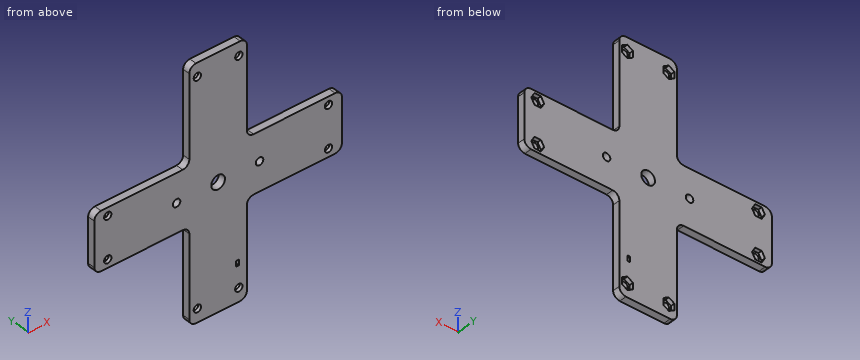
Autodesk Inventor part; units mm, degrees
ref_plane "YZ Plane" through (0, 0, 0) normal (1, 0, 0) x (0, 1, 0)
ref_plane "XZ Plane" through (0, 0, 0) normal (0, 1, 0) x (-1, 0, 0)
ref_plane "XY Plane" through (0, 0, 0) normal (0, 0, 1) x (1, 0, 0)
sketch "Sketch1" plane through (0, 0, 0) normal (0, 1, 0) x (1, 0, 0)
  circle A0 centre (0, 0) radius 2.25
  circle A1 centre (31, 0) radius 2.25
  circle A2 centre (0, 31) radius 2.25
  circle A3 centre (31, 31) radius 2.25
  circle A4 centre (15.5, 15.5) radius 5.125
  line L0 (-6, 37) -> (37, 37)
  line L1 (37, 37) -> (37, -6)
  line L2 (37, -6) -> (-6, -6)
  line L3 (-6, -6) -> (-6, 37)
  line L4 (-6, 37) -> (37, -6) construction
  line L5 (37, 37) -> (-6, -6) construction
  line L6 (-6, -6) -> (37, -6)
  circle A5 centre (0, 98) radius 2.75
  circle A6 centre (31, 98) radius 2.75
  line L7 (-6, 37) -> (37, 37)
  line L8 (37, 37) -> (37, 108)
  line L9 (37, 108) -> (-6, 108)
  line L10 (-6, 108) -> (-6, 37)
  line L11 (15.5, 15.5) -> (22.827, 15.5)
  line L12 (13, 103) -> (18, 103)
  line L13 (15.5, 103) -> (15.5, 96.4439)
  arc A7 (0, 95.25) -> (0, 100.75) centre (0, 98) ccw
  circle A8 centre (-15.5, 15.5) radius 2.7971
  circle A9 centre (46.5, 15.5) radius 2.7971
  line L14 (0, 93.4736) -> (-3.92, 95.7368)
  line L15 (-3.92, 95.7368) -> (-3.92, 100.2632)
  line L16 (-3.92, 100.2632) -> (0, 102.5264)
  line L17 (0, 102.5264) -> (3.92, 100.2632)
  line L18 (3.92, 100.2632) -> (3.92, 95.7368)
  line L19 (3.92, 95.7368) -> (0, 93.4736)
  line L20 (4.17, 100.4076) -> (0, 102.8151)
  line L21 (0, 102.8151) -> (-4.17, 100.4076)
  line L22 (-4.17, 100.4076) -> (-4.17, 95.5924)
  line L23 (-4.17, 95.5924) -> (0, 93.1849)
  line L24 (0, 93.1849) -> (4.17, 95.5924)
  line L25 (4.17, 95.5924) -> (4.17, 100.4076)
  circle A10 centre (31, 98) radius 2.75
  circle A11 centre (31, 98) radius 2.75
  arc A12 (31, 100.75) -> (31, 95.25) centre (31, 98) ccw
  line L26 (31, 93.4736) -> (34.92, 95.7368)
  line L27 (34.92, 95.7368) -> (34.92, 100.2632)
  line L28 (34.92, 100.2632) -> (31, 102.5264)
  line L29 (31, 102.5264) -> (27.08, 100.2632)
  line L30 (27.08, 100.2632) -> (27.08, 95.7368)
  line L31 (27.08, 95.7368) -> (31, 93.4736)
  line L32 (26.83, 100.4076) -> (31, 102.8151)
  line L33 (31, 102.8151) -> (35.17, 100.4076)
  line L34 (35.17, 100.4076) -> (35.17, 95.5924)
  line L35 (35.17, 95.5924) -> (31, 93.1849)
  line L36 (31, 93.1849) -> (26.83, 95.5924)
  line L37 (26.83, 95.5924) -> (26.83, 100.4076)
  line L38 (-64.7368, -3.92) -> (-69.2632, -3.92)
  line L39 (-69.4076, -4.17) -> (-64.5924, -4.17)
  line L40 (-69.2632, -3.92) -> (-71.5264, 0)
  line L41 (-71.8151, 0) -> (-69.4076, -4.17)
  circle A13 centre (-67, 31) radius 2.75
  line L42 (-72, 13) -> (-72, 18)
  line L43 (-69.2632, 27.08) -> (-64.7368, 27.08)
  line L44 (-64.7368, 34.92) -> (-69.2632, 34.92)
  line L45 (-64.5924, 26.83) -> (-69.4076, 26.83)
  circle A14 centre (-67, 31) radius 2.75
  circle A15 centre (-67, 31) radius 2.75
  arc A16 (-69.75, 31) -> (-64.25, 31) centre (-67, 31) ccw
  line L46 (-72, 15.5) -> (-65.4439, 15.5)
  line L47 (-69.2632, 34.92) -> (-71.5264, 31)
  line L48 (-71.8151, 31) -> (-69.4076, 35.17)
  line L49 (-69.4076, 35.17) -> (-64.5924, 35.17)
  line L50 (-71.5264, 31) -> (-69.2632, 27.08)
  line L51 (-69.4076, 26.83) -> (-71.8151, 31)
  line L52 (-62.4736, 0) -> (-64.7368, -3.92)
  line L53 (-64.5924, -4.17) -> (-62.1849, 0)
  circle A17 centre (-67, 0) radius 2.75
  arc A18 (-64.25, 0) -> (-69.75, 0) centre (-67, 0) ccw
  line L54 (-71.5264, 0) -> (-69.2632, 3.92)
  line L55 (-69.4076, 4.17) -> (-71.8151, 0)
  line L56 (-69.2632, 3.92) -> (-64.7368, 3.92)
  line L57 (-64.5924, 4.17) -> (-69.4076, 4.17)
  line L58 (-62.1849, 0) -> (-64.5924, 4.17)
  line L59 (-64.7368, 3.92) -> (-62.4736, 0)
  line L60 (-62.1849, 31) -> (-64.5924, 26.83)
  line L61 (-64.7368, 27.08) -> (-62.4736, 31)
  line L62 (-77, -6) -> (-6, -6)
  line L63 (-62.4736, 31) -> (-64.7368, 34.92)
  line L64 (-64.5924, 35.17) -> (-62.1849, 31)
  line L65 (-77, 37) -> (-77, -6)
  line L66 (-6, 37) -> (-77, 37)
  line L67 (34.92, -64.7368) -> (34.92, -69.2632)
  line L68 (35.17, -69.4076) -> (35.17, -64.5924)
  line L69 (34.92, -69.2632) -> (31, -71.5264)
  line L70 (31, -71.8151) -> (35.17, -69.4076)
  circle A19 centre (0, -67) radius 2.75
  line L71 (18, -72) -> (13, -72)
  line L72 (3.92, -69.2632) -> (3.92, -64.7368)
  line L73 (-3.92, -64.7368) -> (-3.92, -69.2632)
  line L74 (4.17, -64.5924) -> (4.17, -69.4076)
  circle A20 centre (0, -67) radius 2.75
  circle A21 centre (0, -67) radius 2.75
  arc A22 (0, -69.75) -> (0, -64.25) centre (0, -67) ccw
  line L75 (15.5, -72) -> (15.5, -65.4439)
  line L76 (-3.92, -69.2632) -> (0, -71.5264)
  line L77 (0, -71.8151) -> (-4.17, -69.4076)
  line L78 (-4.17, -69.4076) -> (-4.17, -64.5924)
  line L79 (0, -71.5264) -> (3.92, -69.2632)
  line L80 (4.17, -69.4076) -> (0, -71.8151)
  line L81 (31, -62.4736) -> (34.92, -64.7368)
  line L82 (35.17, -64.5924) -> (31, -62.1849)
  circle A23 centre (31, -67) radius 2.75
  arc A24 (31, -64.25) -> (31, -69.75) centre (31, -67) ccw
  line L83 (31, -71.5264) -> (27.08, -69.2632)
  line L84 (26.83, -69.4076) -> (31, -71.8151)
  line L85 (27.08, -69.2632) -> (27.08, -64.7368)
  line L86 (26.83, -64.5924) -> (26.83, -69.4076)
  line L87 (31, -62.1849) -> (26.83, -64.5924)
  line L88 (27.08, -64.7368) -> (31, -62.4736)
  line L89 (0, -62.1849) -> (4.17, -64.5924)
  line L90 (3.92, -64.7368) -> (0, -62.4736)
  line L91 (37, -77) -> (37, -6)
  line L92 (0, -62.4736) -> (-3.92, -64.7368)
  line L93 (-4.17, -64.5924) -> (0, -62.1849)
  line L94 (-6, -77) -> (37, -77)
  line L95 (-6, -6) -> (-6, -77)
  line L96 (95.7368, 34.92) -> (100.2632, 34.92)
  line L97 (100.4076, 35.17) -> (95.5924, 35.17)
  line L98 (100.2632, 34.92) -> (102.5264, 31)
  line L99 (102.8151, 31) -> (100.4076, 35.17)
  circle A25 centre (98, 0) radius 2.75
  line L100 (103, 18) -> (103, 13)
  line L101 (100.2632, 3.92) -> (95.7368, 3.92)
  line L102 (95.7368, -3.92) -> (100.2632, -3.92)
  line L103 (95.5924, 4.17) -> (100.4076, 4.17)
  circle A26 centre (98, 0) radius 2.75
  circle A27 centre (98, 0) radius 2.75
  arc A28 (100.75, 0) -> (95.25, 0) centre (98, 0) ccw
  line L104 (103, 15.5) -> (96.4439, 15.5)
  line L105 (100.2632, -3.92) -> (102.5264, 0)
  line L106 (102.8151, 0) -> (100.4076, -4.17)
  line L107 (100.4076, -4.17) -> (95.5924, -4.17)
  line L108 (102.5264, 0) -> (100.2632, 3.92)
  line L109 (100.4076, 4.17) -> (102.8151, 0)
  line L110 (93.4736, 31) -> (95.7368, 34.92)
  line L111 (95.5924, 35.17) -> (93.1849, 31)
  circle A29 centre (98, 31) radius 2.75
  arc A30 (95.25, 31) -> (100.75, 31) centre (98, 31) ccw
  line L112 (102.5264, 31) -> (100.2632, 27.08)
  line L113 (100.4076, 26.83) -> (102.8151, 31)
  line L114 (100.2632, 27.08) -> (95.7368, 27.08)
  line L115 (95.5924, 26.83) -> (100.4076, 26.83)
  line L116 (93.1849, 31) -> (95.5924, 26.83)
  line L117 (95.7368, 27.08) -> (93.4736, 31)
  line L118 (93.1849, 0) -> (95.5924, 4.17)
  line L119 (95.7368, 3.92) -> (93.4736, 0)
  line L120 (108, 37) -> (37, 37)
  line L121 (93.4736, 0) -> (95.7368, -3.92)
  line L122 (95.5924, -4.17) -> (93.1849, 0)
  line L123 (108, -6) -> (108, 37)
  line L124 (37, -6) -> (108, -6)
  point P0 (37, 37)
  point P1 (37, 37)
  point P2 (-3.5, 98)
  point P3 (34.5, 98)
  point P4 (-67, -3.5)
  point P5 (-67, 34.5)
  point P6 (34.5, -67)
  point P7 (-3.5, -67)
  point P8 (98, 34.5)
  point P9 (98, -3.5)
  point P10 (-6, -6)
  point P11 (-6, -6)
  point P12 (-6, -6)
  point P13 (-6, -6)
  point P14 (-6, -6)
  point P15 (37, 37)
  dimension "d3" = 4.5
  dimension "d5" = 31
  dimension "d6" = 10.25
  dimension "d8" = 43
  dimension "d23" = 5.5
  dimension "d24" = 31
  dimension "d25" = 31
  dimension "d27" = 6
  dimension "d28" = 10
  dimension "d71" = 62
  dimension "d72" = 31
  dimension "d73" = 7.84
  dimension "d74" = 0.25
  dimension "d81" = 82.5
  dimension "d84" = 360
extrude "Extrusion4" add sketch "Sketch1" against normal blind 5.5 contours A0 | A1 | A2 | A3 | L10 L9 L8 L0 | L0 L1 L2 L3 | L3 L62 L65 L66 | L120 L123 L124 L1 | L2 L91 L94 L95 | L14 L15 L16 L17 L18 L19 | L25 L24 L23 L22 L21 L20 | L31 L30 L29 L28 L27 L26 | L32 L33 L34 L35 L36 L37 | L38 L40 L54 L56 L59 L52 | L41 L55 L57 L58 L53 L39 | L50 L47 L44 L63 L61 L43 | L45 L51 L48 L49 L64 L60 | L67 L69 L83 L85 L88 L81 | L70 L84 L86 L87 L82 L68 | L79 L76 L73 L92 L90 L72 | L74 L80 L77 L78 L93 L89 | L96 L98 L112 L114 L117 L110 | L99 L113 L115 L116 L111 L97 | L108 L105 L102 L121 L119 L101 | L103 L109 L106 L107 L122 L118
fillet "Fillet4" radius 5 4 edges at (-6, -2.75, -37) (-6, -2.75, 6) (37, -2.75, 6) (37, -2.75, -37)
fillet "Fillet5" radius 5 8 edges at (37, -2.75, -108) (-6, -2.75, -108) (108, -2.75, 6) (108, -2.75, -37) (37, -2.75, 77) (-6, -2.75, 77) (-77, -2.75, 6) (-77, -2.75, -37)
extrude "Extrusion7" cut sketch "Sketch1" against normal blind 3 contours A5 | A6 | L14 L15 L16 L17 L18 L19 | L25 L24 L23 L22 L21 L20 | L31 L30 L29 L28 L27 L26 | L32 L33 L34 L35 L36 L37 | L38 L40 L54 L56 L59 L52 | L41 L55 L57 L58 L53 L39 | A13 | L50 L47 L44 L63 L61 L43 | L45 L51 L48 L49 L64 L60 | A17 | L67 L69 L83 L85 L88 L81 | L70 L84 L86 L87 L82 L68 | A19 | L79 L76 L73 L92 L90 L72 | L74 L80 L77 L78 L93 L89 | A23 | L96 L98 L112 L114 L117 L110 | L99 L113 L115 L116 L111 L97 | A25 | L108 L105 L102 L121 L119 L101 | L103 L109 L106 L107 L122 L118 | A29
sketch "Sketch6" plane through (0, 0, 0) normal (0, 1, 0) x (1, 0, 0)
  line L0 (31, 78) -> (29, 78)
  line L1 (29, 78) -> (29, 82)
  line L2 (29, 82) -> (31, 82)
  line L3 (31, 82) -> (31, 78)
  line L4 (37, 42) -> (37, 103)
  line L5 (32, 108) -> (-1, 108)
  circle A0 centre (31, 98) radius 2.75
  point P0 (0, 0)
  dimension "d86" = 2
  dimension "d87" = 4
  dimension "d88" = 6
  dimension "d92" = 16
extrude "Extrusion8" cut sketch "Sketch6" against normal through all contours L0 L1 L2 L3
properties part number "motor_holder"
Source: CAD feature listing. Evaluate the final solid. Frame: model axes, mm. Round coordinates to 2 decimals unless told otherwise and drop trailing zeros. Write each loop counter-clockwise with the first axis right and the second up, starting at its lowest first coordinate (ties: lowest second). Pieces come first, ordered by that corner, then holes. Notation, with made-up numbers: (-4, -0.5) - (3, -0.5) arc R19 ccw to (3, 27.5) - close; hole circle Ø7 at (-13.5, 15). An arc over 180 degrees is marked (long way). Use CSV: the item, a comma, the result in double quotes. Start each with the question number.
(1) Cut plane D-D, the plane y = -1.65. Give the number of separate pieces and of enclosed holes in the cut face, and give its area (3 significant figures).
(2) Cut plane A-A, the plane x = -67. Return loops of the section in (y, z).
(3) Cut plane B-B, the plane x = 15.5. Return loops of the section in (y, z) (3 decimals), and give its area (3 significant figures).
(4) Material intervals for probe 1 along Z at (x, y) = (98.5, -1.85); probe 2 along X at (y, z) = (-3.8, -98); probe 3 along X at (y, z) = (-4.3, 0), sorted ascending. Write a range as [from, to].
(5) Cut plane C-C, the plane z = -98. Return loops of the section in (x, y), and give its area (3 significant figures).
(6) First-contact query: pin 1 Ø2 at (x, y) = (37.5, -3.5) entering from -Z; pin 2 Ø1.5 at (x, z) = (-52.5, -24.5) entering from +Y; pin 3 Ø2.5 at (y, z) = (-2, 68) entering from -X; pin 4 Ø6.5 at (x, z) = (0, 67) entering from +Y. Flat tips, straight axial feed; report the tip coordinate or a pass-through.
Geometry says:
1,separate pieces,"1"
1,enclosed holes,"12"
1,area,"13,400 mm²"
2,outline,"(-5.5, -37) - (0, -37) - (0, -35.17) - (-3, -35.17) - (-3, -33.75) - (-5.5, -33.75) - close; (-5.5, -28.25) - (-3, -28.25) - (-3, -26.83) - (0, -26.83) - (0, -4.17) - (-3, -4.17) - (-3, -2.75) - (-5.5, -2.75) - close; (-5.5, 2.75) - (-3, 2.75) - (-3, 4.17) - (0, 4.17) - (0, 6) - (-5.5, 6) - close"
3,outline,"(-5.5, -108) - (0, -108) - (0, -20.625) - (-5.5, -20.625) - close; (-5.5, -10.375) - (0, -10.375) - (0, 77) - (-5.5, 77) - close"
3,area,"961 mm²"
4,probe 1,"[-37, -35.17], [-26.83, -4.17], [4.17, 6]"
4,probe 2,"[-6, -2.75], [2.75, 28.25], [33.75, 37]"
4,probe 3,"[-77, -69.75], [-64.25, 95.25], [100.75, 108]"
5,outline,"(-6, -5.5) - (-2.75, -5.5) - (-2.75, -3) - (-4.17, -3) - (-4.17, 0) - (-6, 0) - close; (2.75, -5.5) - (28.25, -5.5) - (28.25, -3) - (26.83, -3) - (26.83, 0) - (4.17, 0) - (4.17, -3) - (2.75, -3) - close; (33.75, -5.5) - (37, -5.5) - (37, 0) - (35.17, 0) - (35.17, -3) - (33.75, -3) - close"
5,area,"159 mm²"
6,pin 1,"z = -105.18"
6,pin 2,"y = 0"
6,pin 3,"x = -6"
6,pin 4,"y = -3"
